```python
from build123d import *

# Parameters (mm, degrees)
BOSS_EXTRUDE1_DEPTH      = 7.6
BOSS_EXTRUDE1_DEPTH_BACK = 7.6
SKETCH1_R                = 5.5
SKETCH1_R_2              = 3.175
BOSS_EXTRUDE2_START      = 7.6
SKETCH2_R                = 5.5
BOSS_EXTRUDE2_DEPTH      = 2
BOSS_EXTRUDE3_START      = -5.6
SKETCH2_2_R              = 5.5
BOSS_EXTRUDE3_DEPTH      = 2


with BuildPart() as part:
    # Sketch1 → Boss-Extrude1 (new, two sides: drawn at the far end of the back side and taken through both)
    with BuildSketch(Plane(origin=(0, 0, 0), x_dir=(1, 0, 0), z_dir=(0, 1, 0)).offset(-BOSS_EXTRUDE1_DEPTH_BACK)):
        with Locations(Location((0, 0, 0), (0, 0, 270))):
            Circle(SKETCH1_R)
        with Locations(Location((0, 0, 0), (0, 0, 270))):
            Circle(SKETCH1_R_2, mode=Mode.SUBTRACT)
    extrude(amount=BOSS_EXTRUDE1_DEPTH + BOSS_EXTRUDE1_DEPTH_BACK)

    # Sketch2 → Boss-Extrude2 (add)
    with BuildSketch(Plane(origin=(0, 0, 0), x_dir=(1, 0, 0), z_dir=(0, 1, 0)).offset(BOSS_EXTRUDE2_START)):
        with BuildLine():
            Line((-20, 10), (20, 10))
            Line((20, 10), (20, 7.97918472))
            Line((20, 7.97918472), (6.01040764, -6.01040764))
            ThreePointArc((6.01040764, -6.01040764), (0, -8.5), (-6.01040764, -6.01040764))
            Line((-6.01040764, -6.01040764), (-20, 7.97918472))
            Line((-20, 7.97918472), (-20, 10))
        make_face()
        with Locations(Location((0, 0, 0), (0, 0, 270))):
            Circle(SKETCH2_R, mode=Mode.SUBTRACT)
    extrude(amount=-BOSS_EXTRUDE2_DEPTH)

    # Sketch2<2> → Boss-Extrude3 (add)
    with BuildSketch(Plane(origin=(0, 0, 0), x_dir=(1, 0, 0), z_dir=(0, 1, 0)).offset(BOSS_EXTRUDE3_START)):
        with BuildLine():
            Line((-20, 10), (20, 10))
            Line((20, 10), (20, 7.97918472))
            Line((20, 7.97918472), (6.01040764, -6.01040764))
            ThreePointArc((6.01040764, -6.01040764), (0, -8.5), (-6.01040764, -6.01040764))
            Line((-6.01040764, -6.01040764), (-20, 7.97918472))
            Line((-20, 7.97918472), (-20, 10))
        make_face()
        with Locations(Location((0, 0, 0), (0, 0, 270))):
            Circle(SKETCH2_2_R, mode=Mode.SUBTRACT)
    extrude(amount=-BOSS_EXTRUDE3_DEPTH)

    # Fillet1: read off the stored shape, not the designer's step
    # Fillet1 outline → Fillet1 (revolve)
    with BuildSketch(Plane.XY):
        with BuildLine():
            ThreePointArc((5.5, 2.6), (6.378679656, 4.721320344), (8.5, 5.6))
            Line((8.5, 5.6), (5.5, 5.6))
            Line((5.5, 5.6), (5.5, 2.6))
        make_face()
        with BuildLine():
            ThreePointArc((8.5, -5.6), (6.378679656, -4.721320344), (5.5, -2.6))
            Line((5.5, -2.6), (5.5, -5.6))
            Line((5.5, -5.6), (8.5, -5.6))
        make_face()
    revolve(axis=Axis((0, 0, 0), (0, 1, 0)))


solid = part.part
```
The listing builds one solid part. Answer for the finished solid, in the listing's coordinates (mm). Give positions to 0.01 mm unless a question says otherwise; leave off trailing zeros. Order: outer loops, then holes, each group sorted by start corner. A loop starts at its lowest first (then second) coordinate and runs counter-clockwise, first axis right, second up. Notation, with made-up numbers: (52.25, -34.75) - (81.25, -34.75) arc R13 cw to (81.25, -18.75) - close; hole circle Ø6 at (19, 2.25). An arc over 180 degrees is marked (long way). Answer in a Markdown table with one row per item. Add a question column.
Q1. The part is cut by section D-D (x = 17.5). Determine the outline of the cut face in (y, z), then the cut area to 3 significant figures.
Q2. Find the intervals of material crossed by line 1 along Y through (x, z) = (-9.5, -3); line 2 along X through (y, z) = (-0.5, 0) (3 decimals); line 3 along X through (y, z) = (3.5, 0) (3 decimals), in increasing order. Write a range as [from, to].
Q3. The part is cut by section A-A (x = 0). Determine the outline of the cut face in (y, z) (3 decimals).
Q4. For a pull along X with two mould halves and no side action, classify faces 1 (the flat face through (-20, 7, -9)), 2 (the cylindrical face through (1.652, -0.036, 5.246)), 3 (the cylindrical face through (-1.93, -0.11, -2.52)) as released by +X, released by -X, zero draft, split by the parting line, or undercut.
Q5. The part is cut by section C-C (y = -0.5). Determine the outline of the cut face in (x, z) (3 decimals).
Q6. The part is cut by section B-B (z = 0). Determine the outline of the cut face in (x, y) (3 decimals).
Q7. Given P1, Ø6, axis at y = 3.5, z = -6, coming from the +X side; P2, Ø1.5, axis at y = 6, z = 5, coming from the +X side; P3, Ø2, axis at x = -4.5, y = 3, coming from the -Z side, each flat-ended and moving along its own axis, determine where each tip first touches the part or whether it passes through.
Determined:
| question | item | result |
|---|---|---|
| 1 | outline | (-7.6, -10) - (-5.6, -10) - (-5.6, -5.48) - (-7.6, -5.48) - close; (5.6, -10) - (7.6, -10) - (7.6, -5.48) - (5.6, -5.48) - close |
| 1 | area | 18.1 mm² |
| 2 | line 1 | y = [-7.6, -5.6], [5.6, 7.6] |
| 2 | line 2 | x = [-5.5, -3.175], [3.175, 5.5] |
| 2 | line 3 | x = [-5.638, -3.175], [3.175, 5.638] |
| 3 | outline | (-7.6, -10) - (-5.6, -10) - (-5.6, -8.5) arc R3 cw to (-2.6, -5.5) - (2.6, -5.5) arc R3 cw to (5.6, -8.5) - (5.6, -10) - (7.6, -10) - (7.6, -3.175) - (-7.6, -3.175) - close; (-7.6, 3.175) - (7.6, 3.175) - (7.6, 8.5) - (5.6, 8.5) arc R3 cw to (2.6, 5.5) - (-2.6, 5.5) arc R3 cw to (-5.6, 8.5) - (-7.6, 8.5) - close |
| 4 | face 1 | released by -X |
| 4 | face 2 | split by the parting line |
| 4 | face 3 | undercut |
| 5 | outline | circle Ø11 at (0, 0); hole circle Ø6.35 at (0, 0) |
| 6 | outline | (-12.021, -7.6) - (-3.175, -7.6) - (-3.175, 7.6) - (-12.021, 7.6) - (-12.021, 5.6) - (-8.5, 5.6) arc R3 cw to (-5.5, 2.6) - (-5.5, -2.6) arc R3 cw to (-8.5, -5.6) - (-12.021, -5.6) - close; (3.175, -7.6) - (12.021, -7.6) - (12.021, -5.6) - (8.5, -5.6) arc R3 cw to (5.5, -2.6) - (5.5, 2.6) arc R3 cw to (8.5, 5.6) - (12.021, 5.6) - (12.021, 7.6) - (3.175, 7.6) - close |
| 7 | P1 | stops at x = 20 |
| 7 | P2 | stops at x = 7.77 |
| 7 | P3 | stops at z = -4.31 |
